Can you work these out from the model? Positions are in its coordinate system, mm. Coordinates: 2 decimals unless noted, no trailing zeros. Order: outer loops, then holes, each group sorted by start corner. A loop starts at its lowest first (then second) coordinate and runs counter-clockwise, first axis right, second up. Notation, with made-up numbers: M 62,-27 L 97,-27 A15 ccw 97,-16 Z; hole C 28,-37 d6. An arc over 180 degrees is marked long. Answer as a JSON object with one key per item and string values.
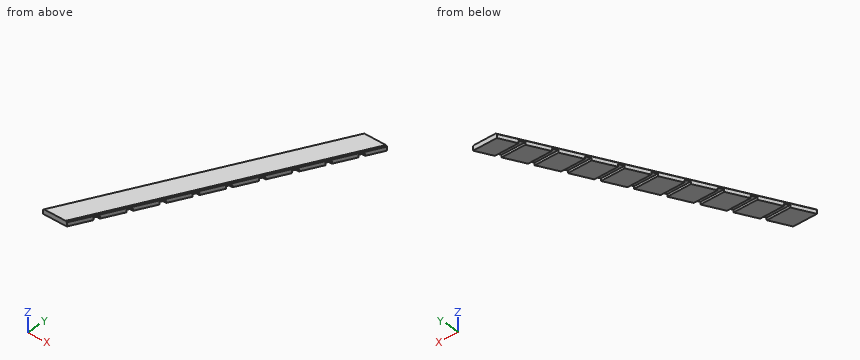
from build123d import *

# Parameters (mm, degrees)
EXTRUDE_1_DEPTH     = 1
SKETCH_2_W          = 34.447182458
SKETCH_2_H          = 1
CUT_EXTRUDE_1_DEPTH = 0.5
CHAMFER_1_SIZE      = 0.2


with BuildPart() as part:
    # Эскиз1 → Бобышка-Вытянуть1 (new body)
    with BuildSketch(Plane.XY):
        Polygon((0, 0), (24.5, 48.3), (19.5, 48.3), (-5, 0), align=None)
    extrude(amount=EXTRUDE_1_DEPTH)

    # Эскиз2 → Вырез-Вытянуть1 (cut)
    with BuildSketch(Plane.XY.offset(1)):
        with Locations((13.095064359, 4.5)):
            Rectangle(SKETCH_2_W, SKETCH_2_H)
        with Locations((13.095064359, 9.5)):
            Rectangle(SKETCH_2_W, SKETCH_2_H)
        with Locations((13.095064359, 14.5)):
            Rectangle(SKETCH_2_W, SKETCH_2_H)
        with Locations((13.095064359, 19.5)):
            Rectangle(SKETCH_2_W, SKETCH_2_H)
        with Locations((13.095064359, 24.5)):
            Rectangle(SKETCH_2_W, SKETCH_2_H)
        with Locations((13.095064359, 29.5)):
            Rectangle(SKETCH_2_W, SKETCH_2_H)
        with Locations((13.095064359, 34.5)):
            Rectangle(SKETCH_2_W, SKETCH_2_H)
        with Locations((13.095064359, 39.5)):
            Rectangle(SKETCH_2_W, SKETCH_2_H)
        with Locations((13.095064359, 44.5)):
            Rectangle(SKETCH_2_W, SKETCH_2_H)
    extrude(amount=-CUT_EXTRUDE_1_DEPTH, mode=Mode.SUBTRACT)


with BuildPart() as body_2:
    # Зеркальное отражение1: mirrored copy
    add(part.part.mirror(Plane.XY.offset(1)))

    # Фаска1
    chamfer_1_edges = [body_2.edges().sort_by_distance(p)[0] for p in [
        (7.25, 24.15, 2),
        (12.25, 24.15, 2),
    ]]
    chamfer(chamfer_1_edges, length=CHAMFER_1_SIZE)


solid = body_2.part
Item 1: I want a section at C-C, the plane x = 4. Write out the boundary of the cut face in (y, z).
Answers follow:
{"outline": "M 7.89,1 L 9,1 L 9,1.5 L 10,1.5 L 10,1 L 14,1 L 14,1.5 L 15,1.5 L 15,1 L 17.74,1 L 17.74,1.8 L 17.3,2 L 8.33,2 L 7.89,1.8 Z"}
Item 2: Please list where these lines run through material, in increasing order: line 1 (Y direction, x = 8.5, z = 1.3); line 2 (Y direction, x = 15.5, z = 1.35).
Answers follow:
{"line 1": "y = 16.76 to 19, 20 to 24, 25 to 26.61", "line 2": "y = 30.56 to 34, 35 to 39, 40 to 40.41"}
Item 3: I want a section at B-B, the plane y = 24.5. Write out the boundary of the cut face in (x, z), plus the area to 3 significant figures.
Answers follow:
{"outline": "M 7.43,1.5 L 12.43,1.5 L 12.43,1.8 L 12.2,2 L 7.65,2 L 7.43,1.8 Z", "area": "2.46 mm^2"}
Item 4: I want a section at A-A, the plane z = 1.25. Give the number of separate pieces and of enclosed holes in the cut face, plus the area to 4 significant figures.
Answers follow:
{"separate pieces": "10", "enclosed holes": "0", "area": "196.5 mm^2"}
Item 5: I'm going to push flat-ended pins straight in: pin 1 (0.8 mm diameter, centred on x = 8, y = 19.5, fed in from -Z); pin 2 (0.6 mm diameter, centred on x = 18, z = 1, fed in from -Y). Where does each tip first touch, or does it pass through?
Answers follow:
{"pin 1": "stops at z = 1.5", "pin 2": "stops at y = 35"}
